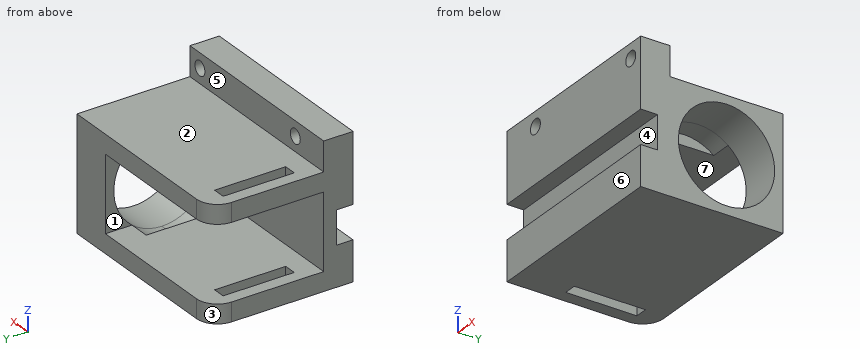
```python
from build123d import *

# Parameters (mm, degrees)
SKETCH_1_W          = 47
SKETCH_1_H          = 34
EXTRUDE_1_DEPTH     = 7
CUT_EXTRUDE_1_DEPTH = 51.46781152378217
HOLE_WIZARD_1_D     = 3.5
EXTRUDE_2_DEPTH     = 27
HOLE_WIZARD_2_D     = 23
HOLE_WIZARD_2_DEPTH = 10
CUT_EXTRUDE_2_DEPTH = 54.04714883949938
CUT_EXTRUDE_START   = -5
SKETCH_11_R         = 11.50000000000001
CUT_EXTRUDE_3_DEPTH = 5
CUT_EXTRUDE_4_DEPTH = 50.36851223198853
FILLET_1_R          = 5


with BuildPart() as part:
    # 草图1 → 凸台-拉伸1 (new body)
    with BuildSketch(Plane(origin=(0, 0, 0), x_dir=(1, 0, 0), z_dir=(0, 1, 0))):
        Rectangle(SKETCH_1_W, SKETCH_1_H)
    extrude(amount=EXTRUDE_1_DEPTH)

    # 草图2 → 切除-拉伸1 (cut, through all)
    with BuildSketch(Plane(origin=(23.500000000000007, 0, 0), x_dir=(0, 0, -1), z_dir=(1, 0, 0))):
        Polygon((-0.4999999999999987, 4), (-0.4999999999999987, 0), (3.5, 0), (7.5, 0), (7.500000000000002, 4), align=None)
    extrude(amount=-CUT_EXTRUDE_1_DEPTH, mode=Mode.SUBTRACT)

    # 孔1 (through all)
    with Locations(Plane(origin=(0, 7, 0), x_dir=(1, 0, 0), z_dir=(0, 1, 0))):
        with Locations((-13.5, -13.5), (20, -13.5)):
            Hole(HOLE_WIZARD_1_D / 2)

    # 草图6 → 凸台-拉伸2 (add)
    with BuildSketch(Plane(origin=(0, 7, 0), x_dir=(1, 0, 0), z_dir=(0, 1, 0))):
        Polygon((-23.499999999999993, -10.000000000000009), (23.500000000000007, -10.000000000000002), (23.500000000000007, 17), (-23.499999999999993, 17), align=None)
    extrude(amount=EXTRUDE_2_DEPTH)

    # 孔2
    with Locations(Plane(origin=(23.500000000000007, 0, 0), x_dir=(0, 0, -1), z_dir=(1, 0, 0))):
        with Locations((3.5, 20.5)):
            Hole(HOLE_WIZARD_2_D / 2, depth=HOLE_WIZARD_2_DEPTH)

    # 草图10 → 切除-拉伸2 (cut, through all)
    with BuildSketch(Plane(origin=(13.500000000000007, 0, 0), x_dir=(0, 0, -1), z_dir=(1, 0, 0))):
        Polygon((-5.5000000000000036, 34.00000000000001), (12.499999999999998, 34.00000000000001), (12.499999999999998, 7.000000000000013), (-5.5, 7.000000000000013), align=None)
    extrude(amount=-CUT_EXTRUDE_2_DEPTH, mode=Mode.SUBTRACT)

    # 草图11 → 切除-拉伸3 (cut)
    with BuildSketch(Plane(origin=(13.500000000000007, 0, 0), x_dir=(0, 0, -1), z_dir=(1, 0, 0)).offset(CUT_EXTRUDE_START)):
        with Locations((3.500000000000003, 20.500000000000004)):
            Circle(SKETCH_11_R)
    extrude(amount=CUT_EXTRUDE_3_DEPTH, mode=Mode.SUBTRACT)

    # 草图12 → 切除-拉伸4 (cut, through all)
    with BuildSketch(Plane.XY.offset(10.000000000000005)):
        Polygon((-20.499999999999993, 29), (-17.499999999999996, 29), (-17.499999999999993, 12), (-20.49999999999999, 12), align=None)
    extrude(amount=-CUT_EXTRUDE_4_DEPTH, mode=Mode.SUBTRACT)

    # 圆角1
    fillet_1_edges = [part.edges().sort_by_distance(p)[0] for p in [
        (-23.499999999999993, 34, -14.75),
        (-23.499999999999993, 34, 7.750000000000007),
    ]]
    fillet(fillet_1_edges, radius=FILLET_1_R)


solid = part.part
```
Source: CAD feature listing. Evaluate the final solid. Frame: model axes, mm. Face numbers are marked on the shaded views. A direction names the side the tool comes from. Coordinates: 2 decimals unless noted, no trailing zeros. Order: outer loops, then holes, each group sorted by start corner. A loop starts at its lowest first (then second) coordinate and runs counter-clockwise, first axis right, second up. Notation, with made-up numbers: (40.5, 7.5) - (52.5, 7.5) arc R18 cw to (52.5, 12.5) - close; hole circle Ø6 at (-29.75, -11.5). An arc over 180 degrees is marked (long way). One line per item, written item: value.
1) Contact query for flat-ended pins moving along their axis: pin 1 (6 mm diameter, centred on x = -11.5, y = 15.5, fed in from +Z); pin 2 (3 mm diameter, centred on y = 29.5, z = -6, fed in from -X); pin 3 (1 mm diameter, centred on x = 13, z = 12, fed in from +Y); pin 4 (3 mm diameter, centred on x = -8.5, z = -2, fed in from -Y). Output: stop coordinate, or through.
Computed values:
pin 1: stops at z = 10
pin 2: passes through
pin 3: stops at y = 7
pin 4: stops at y = 4
2) Mould query, pull axis Z, two halves, no side actions, for the marked faces 1, 2, 3 and 4. Classes: released by +Z, released by -Z, zero draft, split by the parting line, or undercut.
Computed values:
face 1: undercut
face 2: released by +Z
face 3: zero draft
face 4: undercut
3) Ray query, line 1 (Z direction, x = 20, y = 3.5); line 2 (X direction, y = 3.75, z = 13.5); line 3 (Z direction, x = 19, y = 20). Return the intervals inside material, ascending. Write a range as [from, to].
Computed values:
line 1: z = [-17, -7.5], [0.5, 11.75], [15.25, 17]
line 2: x = [-23.5, -15.25], [-11.75, 18.25], [21.75, 23.5]
line 3: z = [-17, -14.99], [7.99, 10]
4) Cut plane D-D on y = 31. Output: boundary loops of the cut face in (x, z), plus the area to 3 significant figures.
Computed values:
outline: (-23.08, -17) - (23.5, -17) - (23.5, -8.19) - (13.5, -8.19) - (13.5, -12.5) - (-23.08, -12.5) - close; (-23.08, 5.5) - (13.5, 5.5) - (13.5, 1.19) - (23.5, 1.19) - (23.5, 10) - (-23.08, 10) - close
area: 505 mm^2
5) Cut plane B-B on z = 13.5. Output: boundary loops of the cut face in (x, y).
Computed values:
outline: (-23.5, 0) - (-15.25, 0) - (-15.25, 7) - (-23.5, 7) - close; (-11.75, 0) - (18.25, 0) - (18.25, 7) - (-11.75, 7) - close; (21.75, 0) - (23.5, 0) - (23.5, 7) - (21.75, 7) - close
6) Reachability of the marked faces 5, 6 and 7 from +Z, -Z, +X, -X, +Y, -Y: full face, straight path, thin tool, end or side. Return the list, or none.
Computed values:
face 5: +Z, +X, -X, +Y
face 6: +Z, -Z, +X, -X, -Y
face 7: -X, +Y
7) Cut plane A-A on x = 20. Output: boundary loops of the cut face in (y, z).
Computed values:
outline: (0, -17) - (34, -17) - (34, 10) - (7, 10) - (7, 11.75) - (0, 11.75) - (0, 0.5) - (4, 0.5) - (4, -7.5) - (0, -7.5) - close; (0, 15.25) - (7, 15.25) - (7, 17) - (0, 17) - close; hole circle Ø23 at (20.5, -3.5)
8) Cut plane C-C on z = -3.5. Output: boundary loops of the cut face in (x, y).
Computed values:
outline: (-23.5, 4) - (23.5, 4) - (23.5, 9) - (13.5, 9) - (13.5, 7) - (-23.5, 7) - close; (13.5, 32) - (23.5, 32) - (23.5, 34) - (13.5, 34) - close
